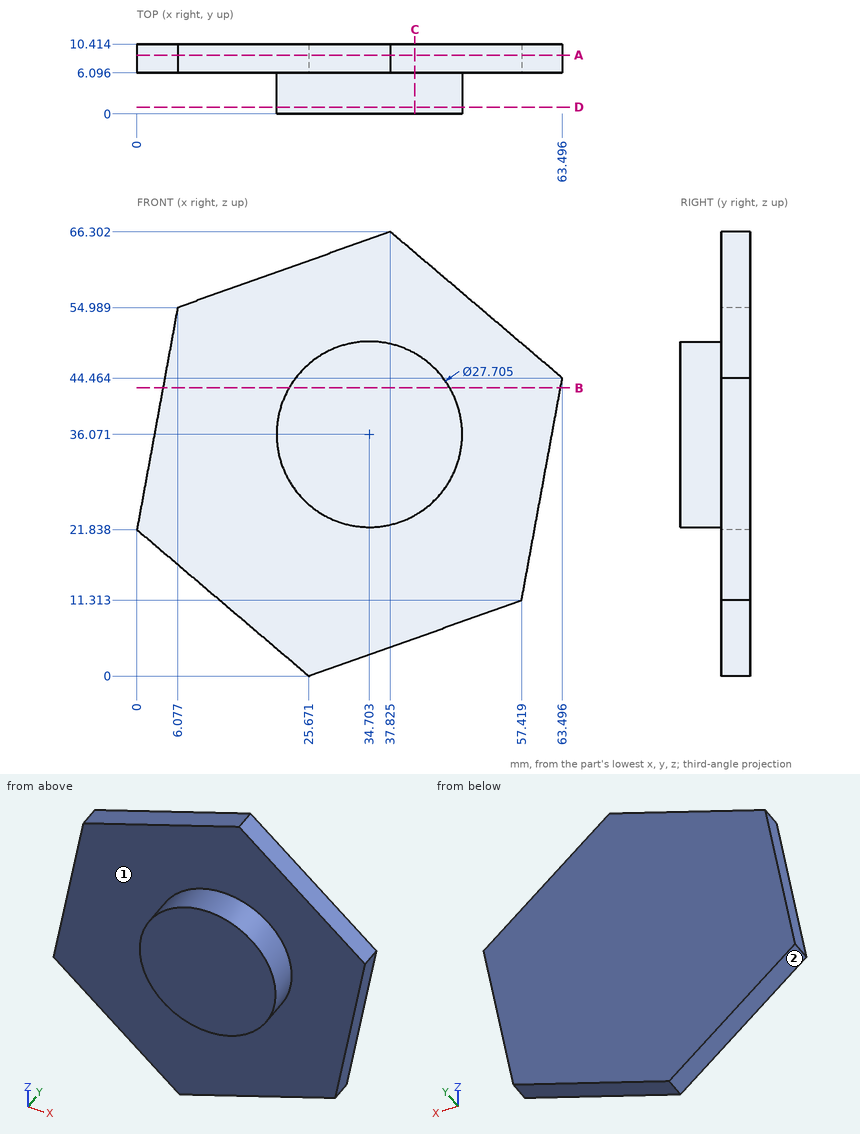
Source: three-view drawing plus pictorial views. Frame: mm from the lowest corner of the part. A direction names the side the tool comes from. Give positions to 0.01 mm unless a question says otherwise; leave off trailing zeros. Order: outer loops, then holes, each group sorted by start corner. A loop starts at its lowest first (then second) coordinate and runs counter-clockwise, first axis right, second up. Notation, with made-up numbers: (89.25, 78) -> (144.25, 78) arc R17 cw to (144.25, 94) -> close; hole circle Ø10 at (-39, 36.25). An arc over 180 degrees is marked (long way). Use a Markdown table: item, result.
Q1. Access query for the marked faces 1 and 2. Directions: +Z, -Z, +X, -X, +Y, -Y. A direction counts if a zero-diameter tool reaches every point of the face in a straight line with its end or side. Return the directions, or none.
A:
| item | result |
|---|---|
| face 1 | -Y |
| face 2 | -Z, -X, +Y, -Y |
Q2. Section B-B (z = 43). Return the cut outline in (x, y).
A:
| item | result |
|---|---|
| outline | (3.88, 6.1) -> (22.71, 6.1) -> (22.71, 0) -> (46.7, 0) -> (46.7, 6.1) -> (63.23, 6.1) -> (63.23, 10.41) -> (3.88, 10.41) -> close |
Q3. Material intervals for line 1 (Y direction, x = 41.5, z = 53); line 2 (X direction, y = 9.5, z = 20.5) (1 decimal); line 3 (Z direction, x = 50.5, y = 9.25) (1 decimal), sorted ascending. Write a range as [from, to].
A:
| item | result |
|---|---|
| line 1 | [6.1, 10.41] |
| line 2 | [1.6, 59.1] |
| line 3 | [8.8, 55.5] |
Q4. Section A-A (y = 8.75). Return the cut outline in (x, z) (1 decimal), and give its area (3 significant figures).
A:
| item | result |
|---|---|
| outline | (0, 21.8) -> (25.7, 0) -> (57.4, 11.3) -> (63.5, 44.5) -> (37.8, 66.3) -> (6.1, 55) -> close |
| area | 2,950 mm^2 |
Q5. Section C-C (x = 41.5). Return the cut outline in (y, z) (1 decimal).
A:
| item | result |
|---|---|
| outline | (0, 24) -> (6.1, 24) -> (6.1, 5.6) -> (10.4, 5.6) -> (10.4, 63.2) -> (6.1, 63.2) -> (6.1, 48.1) -> (0, 48.1) -> close |
Q6. Section D-D (y = 1). Return the cut outline in (x, z) (1 decimal), and give its area (3 significant figures).
A:
| item | result |
|---|---|
| outline | circle Ø27.7 at (34.7, 36.1) |
| area | 603 mm^2 |
Q7. First-contact query: P1, Ø6, axis at y = 4, z = 52.5, coming from the +X side; P2, Ø3, axis at y = 6.5, z = 9, coming from the -X side; P3, Ø4, axis at x = 36.5, z = 53, coming from the -Y side. Flat tips, straight axial feed; report the tip coordinate or a pass-through.
A:
| item | result |
|---|---|
| P1 | x = 56.57 |
| P2 | x = 13.33 |
| P3 | y = 6.1 |
